from build123d import *

# Parameters (mm, degrees)
SKETCH1_R           = 57
BOSS_EXTRUDE1_DEPTH = 186
SKETCH2_R           = 31.83061868
CUT_EXTRUDE1_DEPTH  = 10
FILLET1_R           = 10


with BuildPart() as part:
    # Sketch1 → Boss-Extrude1 (new body)
    with BuildSketch(Plane.XY):
        with Locations(Location((0, 0, 0), (0, 0, 180))):
            Circle(SKETCH1_R)
    extrude(amount=BOSS_EXTRUDE1_DEPTH)

    # Sketch2 → Cut-Extrude1 (cut)
    with BuildSketch(Plane(origin=(0, 0, 0), x_dir=(-1, 0, 0), z_dir=(0, 0, -1))):
        Circle(SKETCH2_R)
    extrude(amount=-CUT_EXTRUDE1_DEPTH, mode=Mode.SUBTRACT)

    # Fillet1
    fillet1_edges = [part.edges().sort_by_distance(p)[0] for p in [
        (31.83061868, 0, 10),
    ]]
    fillet(fillet1_edges, radius=FILLET1_R - 0.0001)  # a hair under: the kernel refuses the full size


solid = part.part
Could you check a few things on this model? Use its own coordinates, in mm. Give positions to 0.01 mm unless a question says otherwise; leave off trailing zeros. Write each loop counter-clockwise with the first axis right and the second up, starting at its lowest first coordinate (ties: lowest second). Pieces come first, ordered by that corner, then holes. Notation, with made-up numbers: (19.5, 53) -> (28.5, 53) arc R21 ccw to (28.5, 90) -> close; hole circle Ø10 at (50, 30.5). An arc over 180 degrees is marked (long way). Answer as a JSON object with one key per item and string values.
Q1. Suppose I cut it at D-D on y = -48. Write out the boundary of the cut face in (x, z).
Taken from the geometry:
{"outline": "(-30.74, 0) -> (30.74, 0) -> (30.74, 186) -> (-30.74, 186) -> close"}
Q2. Please list where these lines run through material, in increasing order: L1, parallel to Y at x = 0, z = 0.05; L2, parallel to X at y = -3, z = 177.5; L3, parallel to X at y = 13, z = 154.
Taken from the geometry:
{"L1": "y = -57 to -31.83, 31.83 to 57", "L2": "x = -56.92 to 56.92", "L3": "x = -55.5 to 55.5"}
Q3. We'd pull the mould along Y, two halves only. Please class faces 1 (the flat face through (-25, 25, 0)), 2 (the flat face through (0, 0, 10)), 3 (the cylindrical face through (12.356, 55.645, 91.698)): released by +Y, released by -Y, zero draft, split by the parting line, or undercut.
Taken from the geometry:
{"face 1": "zero draft", "face 2": "undercut", "face 3": "split by the parting line"}
Q4. Will these pins go through, and if not, where does the flat tip stop? pin 1 Ø8 at (y, z) = (-11.5, 107) entering from +X; pin 2 Ø2 at (x, z) = (45, 114.5) entering from +Y; pin 3 Ø3 at (x, z) = (25, 150) entering from -Y.
Taken from the geometry:
{"pin 1": "stops at x = 56.5", "pin 2": "stops at y = 36.24", "pin 3": "stops at y = -51.93"}
Q5. Suppose I cut it at C-C on z = 77. Write out the boundary of the cut face in (x, y).
Taken from the geometry:
{"outline": "circle Ø114 at (0, 0)"}
